from build123d import *

# Parameters (mm, degrees)
F1_DEPTH = 5
F3_DEPTH = 11
F2_W     = 1
F2_H     = 7
F4_DEPTH = 6
F5_D     = 3


with BuildPart() as f1:
    # F0 (on Top) → F1 (new body)
    with BuildSketch(Plane.XY):
        Polygon((8.783761, 49.804577), (-50.216239, 49.804577), (-50.216239, -22.195423), (11.783761, -22.195423), (11.783761, 36.804577), (8.783761, 36.804577), align=None)
    extrude(amount=F1_DEPTH)

    # F2 (on face) → F3 (join)
    with BuildSketch(Plane.XY.offset(5)):
        Polygon((-37.216239, 35.304577), (-37.216239, 13.804577), (-37.216239, -11.695423), (-36.216239, -11.695423), (-36.216239, 35.304577), align=None)
        Polygon((-33.716239, -11.695423), (-33.716239, 35.304577), (-34.716239, 35.304577), (-34.716239, 13.804577), (-34.716239, -11.695423), align=None)
        Polygon((-31.216239, -11.695423), (-31.216239, 35.304577), (-32.216239, 35.304577), (-32.216239, 13.804577), (-32.216239, -11.695423), align=None)
        Polygon((-28.716239, -11.695423), (-28.716239, 35.304577), (-29.716239, 35.304577), (-29.716239, 13.804577), (-29.716239, -11.695423), align=None)
        Polygon((-26.216239, -11.695423), (-26.216239, 35.304577), (-27.216239, 35.304577), (-27.216239, 13.804577), (-27.216239, -11.695423), align=None)
        Polygon((-23.716239, -11.695423), (-23.716239, 35.304577), (-24.716239, 35.304577), (-24.716239, 13.804577), (-24.716239, -11.695423), align=None)
        Polygon((-21.216239, -11.695423), (-21.216239, 35.304577), (-22.216239, 35.304577), (-22.216239, 13.804577), (-22.216239, -11.695423), align=None)
        Polygon((-19.716239, -11.695423), (-18.716239, -11.695423), (-18.716239, 35.304577), (-19.716239, 35.304577), (-19.716239, 13.804577), align=None)
        Polygon((-16.216239, -11.695423), (-16.216239, 35.304577), (-17.216239, 35.304577), (-17.216239, 13.804577), (-17.216239, -11.695423), align=None)
        Polygon((-13.716239, -11.695423), (-13.716239, 35.304577), (-14.716239, 35.304577), (-14.716239, 13.804577), (-14.716239, -11.695423), align=None)
        Polygon((-11.216239, -11.695423), (-11.216239, 35.304577), (-12.216239, 35.304577), (-12.216239, 13.804577), (-12.216239, -11.695423), align=None)
        Polygon((-8.716239, -11.695423), (-8.716239, 35.304577), (-9.716239, 35.304577), (-9.716239, 13.804577), (-9.716239, -11.695423), align=None)
        Polygon((-6.216239, -11.695423), (-6.216239, 35.304577), (-7.216239, 35.304577), (-7.216239, 13.804577), (-7.216239, -11.695423), align=None)
        Polygon((-3.716239, -11.695423), (-3.716239, 35.304577), (-4.716239, 35.304577), (-4.716239, 13.804577), (-4.716239, -11.695423), align=None)
        Polygon((-1.216239, -11.695423), (-1.216239, 35.304577), (-2.216239, 35.304577), (-2.216239, 13.804577), (-2.216239, -11.695423), align=None)
        Polygon((1.283761, -11.695423), (1.283761, 35.304577), (0.283761, 35.304577), (0.283761, 13.804577), (0.283761, -11.695423), align=None)
        Polygon((3.783761, -11.695423), (3.783761, 35.304577), (2.783761, 35.304577), (2.783761, 13.804577), (2.783761, -11.695423), align=None)
    extrude(amount=F3_DEPTH)

    # F2 (on face) → F4 (join)
    with BuildSketch(Plane.XY.offset(5)):
        with Locations((-36.716239, 38.804577)):
            Rectangle(F2_W, F2_H)
        with Locations((-34.216239, 38.804577)):
            Rectangle(F2_W, F2_H)
        with Locations((-31.716239, 38.804577)):
            Rectangle(F2_W, F2_H)
        with Locations((-29.216239, 38.804577)):
            Rectangle(F2_W, F2_H)
        with Locations((-26.716239, 38.804577)):
            Rectangle(F2_W, F2_H)
        with Locations((-24.216239, 38.804577)):
            Rectangle(F2_W, F2_H)
        with Locations((-21.716239, 38.804577)):
            Rectangle(F2_W, F2_H)
        with Locations((-19.216239, 38.804577)):
            Rectangle(F2_W, F2_H)
        with Locations((-16.716239, 38.804577)):
            Rectangle(F2_W, F2_H)
        with Locations((-14.216239, 38.804577)):
            Rectangle(F2_W, F2_H)
        with Locations((-11.716239, 38.804577)):
            Rectangle(F2_W, F2_H)
        with Locations((-9.216239, 38.804577)):
            Rectangle(F2_W, F2_H)
        with Locations((-6.716239, 38.804577)):
            Rectangle(F2_W, F2_H)
        with Locations((-4.216239, 38.804577)):
            Rectangle(F2_W, F2_H)
        with Locations((-1.716239, 38.804577)):
            Rectangle(F2_W, F2_H)
        with Locations((0.783761, 38.804577)):
            Rectangle(F2_W, F2_H)
        with Locations((3.283761, 38.804577)):
            Rectangle(F2_W, F2_H)
        with Locations((3.283761, -15.195423)):
            Rectangle(F2_W, F2_H)
        with Locations((0.783761, -15.195423)):
            Rectangle(F2_W, F2_H)
        with Locations((-1.716239, -15.195423)):
            Rectangle(F2_W, F2_H)
        with Locations((-4.216239, -15.195423)):
            Rectangle(F2_W, F2_H)
        with Locations((-6.716239, -15.195423)):
            Rectangle(F2_W, F2_H)
        with Locations((-9.216239, -15.195423)):
            Rectangle(F2_W, F2_H)
        with Locations((-11.716239, -15.195423)):
            Rectangle(F2_W, F2_H)
        with Locations((-14.216239, -15.195423)):
            Rectangle(F2_W, F2_H)
        with Locations((-16.716239, -15.195423)):
            Rectangle(F2_W, F2_H)
        Polygon((-19.716239, -18.695423), (-19.216239, -18.695423), (-18.716239, -18.695423), (-18.716239, -11.695423), (-19.716239, -11.695423), align=None)
        with Locations((-21.716239, -15.195423)):
            Rectangle(F2_W, F2_H)
        with Locations((-24.216239, -15.195423)):
            Rectangle(F2_W, F2_H)
        with Locations((-26.716239, -15.195423)):
            Rectangle(F2_W, F2_H)
        with Locations((-29.216239, -15.195423)):
            Rectangle(F2_W, F2_H)
        with Locations((-31.716239, -15.195423)):
            Rectangle(F2_W, F2_H)
        with Locations((-34.216239, -15.195423)):
            Rectangle(F2_W, F2_H)
        with Locations((-36.716239, -15.195423)):
            Rectangle(F2_W, F2_H)
    extrude(amount=F4_DEPTH)

    # F5 (through all)
    with Locations(Plane.XY.offset(5)):
        with Locations((-40.716239, 27.304577), (7.283761, 27.304577), (7.283761, -10.695423), (-40.716239, -10.695423)):
            Hole(F5_D / 2)


solid = f1.part
Geometry: final body of the model. Coordinates: model frame, mm. A direction names the side the tool comes from. Round coordinates to 2 decimals unless told otherwise and drop trailing zeros. Loops run counter-clockwise (first coordinate to the right, second up) from the corner with the lowest first, then second, coordinate; pieces in that order, holes last. Notation, with made-up numbers: M 71.25,20.25 L 90.25,20.25 A30 cw 90.25,49.25 Z; hole C 78.5,-10.5 d7. An arc over 180 degrees is marked long. Put each result on its own line as item: value. Start each with the question number.
(1) Section query B-B (z = 1.75). Return loops of the section in (x, y).
(2) Section query A-A (x = 7.5). Return loops of the section in (y, z).
(3) Contact query for flat-ended pins moving along their axis: pin 1 Ø0.5 at (x, z) = (-16.5, 13) entering from +Y; pin 2 Ø6 at (x, z) = (3.5, 13) entering from -Y; pin 3 Ø0.5 at (x, z) = (-12, 8.5) entering from +Y. Output: stop coordinate, or through.
(4) Material intervals for line 1 along Z through (x, y) = (-25, 4); line 2 along Y through (x, z) = (-14, 11.75), sorted ascending. Write a range as [from, to].
(5) Draft query along Y for faces 1 (the face through (-16.216, 11, 10)), 2 (the face through (-40.39, 25.84, 2.47)), 3 (the face through (-20, 49.805, 2)). Return one class per face: +Y half, -Y half, draft (parallel to the pull), parting line (faces both ways), or undercut.
(6) Set-up query: faces 4 (the face through (7.61, -12.16, 2.47)), 5 (the face through (-19.716, 12, 10)). Return all of +Z, -Z, +X, -X, +Y, -Y with unobstructed straight access to the full face (end or side cutting, diameter ignored); none if empty.
(7) Section query C-C (y = 44.5). Return loops of the section in (x, z), then the cut area to 3 significant figures.
(8) Section query D-D (z = 9.5). State how many separate pieces and enclosed holes the cut face has, then the cut area to 3 significant figures.
Findings below:
1. outline: M -50.22,-22.2 L 11.78,-22.2 L 11.78,36.8 L 8.78,36.8 L 8.78,49.8 L -50.22,49.8 Z; hole C -40.72,-10.7 d3; hole C -40.72,27.3 d3; hole C 7.28,-10.7 d3; hole C 7.28,27.3 d3
2. outline: M -22.2,0 L -12.18,0 L -12.18,5 L -22.2,5 Z; M -9.21,0 L 25.82,0 L 25.82,5 L -9.21,5 Z; M 28.79,0 L 49.8,0 L 49.8,5 L 28.79,5 Z
3. pin 1: stops at y = 35.3
3. pin 2: stops at y = -18.7
3. pin 3: stops at y = 42.3
4. line 1: z = [0, 5]
4. line 2: y = [-11.7, 35.3]
5. face 1: draft
5. face 2: undercut
5. face 3: +Y half
6. face 4: +Z, -Z
6. face 5: +Z, +Y, -Y
7. outline: M -50.22,0 L 8.78,0 L 8.78,5 L -50.22,5 Z
7. area: 295 mm2
8. separate pieces: 17
8. enclosed holes: 0
8. area: 1,040 mm2
